The figure shows three views and two pictorial views of one solid part (mm, origin at its lowest corner). Answer the questions. A direction names the side the tool comes from. Give positions to 0.01 mm unless a question says otherwise; leave off trailing zeros. Loops run counter-clockwise (first coordinate to the right, second up) from the corner with the lowest first, then second, coordinate; pieces in that order, holes last. Notation, with made-up numbers: M 7,-8 L 43,-8 A26 cw 43,16 Z; hole C 35.5,27 d10. An arc over 180 degrees is marked long. One line per item, written item: value. Start each with the question number.
Q1. Consider L1, parallel to Y at x = 16, z = 0.65; L2, parallel to Y at x = 17.5, z = 3.95 (1 decimal); L3, parallel to X at y = 48.5, z = 4.05. Determine where each line is inside the solid, lowest interval first.
Q2. A cutting plane is placed at A-A, the plane y = 50. Determine the outline of the cut face in (x, z).
Q3. A cutting plane is placed at C-C, the plane x = 16. Determine the outline of the cut face in (y, z), and give its area (3 significant figures).
Q4. A cutting plane is placed at D-D, the plane y = 78. Determine the outline of the cut face in (x, z), and give its area (3 significant figures).
Q5. A cutting plane is placed at B-B, the plane z = 3.1. Determine the outline of the cut face in (x, y), and give its area (3 significant figures).
Q6. For the marked faces 1 and 2, determine the directions among +Z, -Z, +X, -X, +Y, -Y from which every point of the face is accessible in a straight line to the end or side of a thin tool.
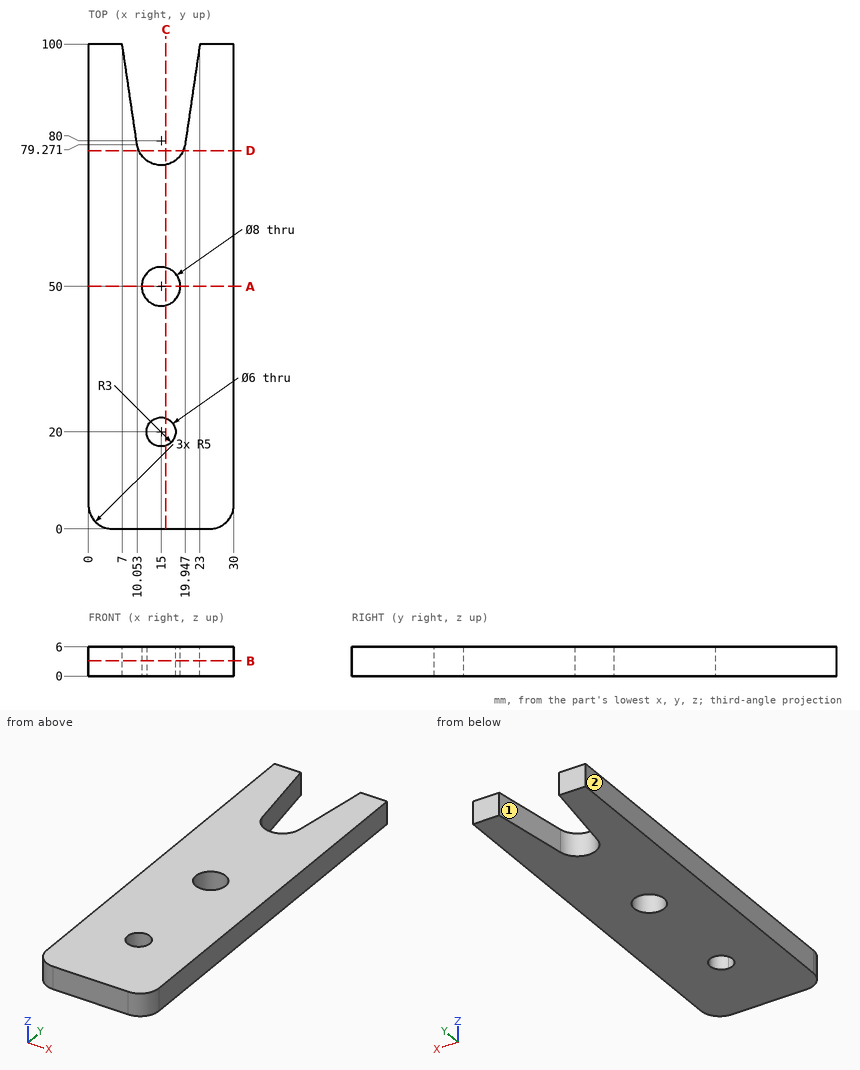
Answer block:
1. L1: 0 to 17.17, 22.83 to 46.13, 53.87 to 75.1
1. L2: 0 to 18.3, 21.7 to 46.9, 53.1 to 75.7
1. L3: 0 to 11.29, 18.71 to 30
2. outline: M 0,0 L 11,0 L 11,6 L 0,6 Z; M 19,0 L 30,0 L 30,6 L 19,6 Z
3. outline: M 0,0 L 17.17,0 L 17.17,6 L 0,6 Z; M 22.83,0 L 46.13,0 L 46.13,6 L 22.83,6 Z; M 53.87,0 L 75.1,0 L 75.1,6 L 53.87,6 Z
3. area: 370 mm^2
4. outline: M 0,0 L 10.42,0 L 10.42,6 L 0,6 Z; M 19.58,0 L 30,0 L 30,6 L 19.58,6 Z
4. area: 125 mm^2
5. outline: M 0,5 A5 ccw 5,0 L 25,0 A5 ccw 30,5 L 30,100 L 23,100 L 19.95,79.27 A5 cw 10.05,79.27 L 7,100 L 0,100 Z; hole C 15,50 d8; hole M 15,17 A3 ccw 18,20 A3 ccw long Z
5. area: 2,610 mm^2
6. face 1: +Z, -Z, +Y
6. face 2: +Z, -Z, -X, +Y, -Y
